```python
from build123d import *

# Parameters (mm, degrees)
ESQUISSE1_W                                    = 100
ESQUISSE1_H                                    = 100
ESQUISSE1_W_2                                  = 56.4
ESQUISSE1_H_2                                  = 56.4
BOSS_EXTRU_1_DEPTH                             = 10
CONG_1_R                                       = 3.2
BOSS_EXTRU_2_START                             = 10
ESQUISSE3_R                                    = 40
BOSS_EXTRU_2_DEPTH                             = 10
ESQUISSE4_OUTSIDE_W                            = 130.566
ESQUISSE4_OUTSIDE_H                            = 130.566
ESQUISSE4_OUTSIDE_R                            = 43
ENL_V_MAT_EXTRU_2_DEPTH                        = 0.5
ESQUISSE5_W                                    = 61.6
ESQUISSE5_H                                    = 61.6
ENL_V_MAT_EXTRU_3_DEPTH                        = 9
ESQUISSE6_W                                    = 61.6
ESQUISSE6_H                                    = 61.6
BOSS_EXTRU_3_DEPTH                             = 1
ESQUISSE12_W                                   = 100
ESQUISSE12_H                                   = 9.5
BOSS_EXTRU_5_DEPTH                             = 20
FRAISAGE_POUR_VIS_T_TE_FRAIS_E_M61_D           = 6.6
FRAISAGE_POUR_VIS_T_TE_FRAIS_E_M61_CSINK_D     = 12.6
FRAISAGE_POUR_VIS_T_TE_FRAIS_E_M61_CSINK_ANGLE = 90
ESQUISSE16_W                                   = 2
ESQUISSE16_H                                   = 10
ENL_V_MAT_EXTRU_4_DEPTH                        = 8
CONG_3_R                                       = 3.5
ESQUISSE17_W                                   = 10
ESQUISSE17_H                                   = 5
ENL_V_MAT_EXTRU_5_DEPTH                        = 89.317608663
CONG_4_R                                       = 3.5
CONG_5_R                                       = 3.3
CONG_6_R                                       = 4


with BuildPart() as part:
    # Esquisse1 → Boss.-Extru.1 (new body)
    with BuildSketch(Plane.XY):
        Rectangle(ESQUISSE1_W, ESQUISSE1_H)
        Rectangle(ESQUISSE1_W_2, ESQUISSE1_H_2, mode=Mode.SUBTRACT)
    extrude(amount=BOSS_EXTRU_1_DEPTH)

    # Congé1
    cong_1_edges = [part.edges().sort_by_distance(p)[0] for p in [
        (-28.2, 28.2, 5),
        (-28.2, -28.2, 5),
        (28.2, -28.2, 5),
        (28.2, 28.2, 5),
    ]]
    fillet(cong_1_edges, radius=CONG_1_R)

    # Esquisse3 → Boss.-Extru.2 (add)
    with BuildSketch(Plane.XY.offset(10).offset(BOSS_EXTRU_2_START)):
        Circle(ESQUISSE3_R)
        with BuildLine():
            Line((-28.2, 25), (-28.2, -25))
            ThreePointArc((-28.2, -25), (-27.2627417, -27.2627417), (-25, -28.2))
            Line((-25, -28.2), (25, -28.2))
            ThreePointArc((25, -28.2), (27.2627417, -27.2627417), (28.2, -25))
            Line((28.2, -25), (28.2, 25))
            ThreePointArc((28.2, 25), (27.2627417, 27.2627417), (25, 28.2))
            Line((25, 28.2), (-25, 28.2))
            ThreePointArc((-25, 28.2), (-27.2627417, 27.2627417), (-28.2, 25))
        make_face(mode=Mode.SUBTRACT)
    extrude(amount=-BOSS_EXTRU_2_DEPTH)

    # Esquisse4 outside → Enlèv. mat.-Extru.2 (cut)
    with BuildSketch(Plane.XY.offset(10)):
        Rectangle(ESQUISSE4_OUTSIDE_W, ESQUISSE4_OUTSIDE_H)
        Circle(ESQUISSE4_OUTSIDE_R, mode=Mode.SUBTRACT)
    extrude(amount=-ENL_V_MAT_EXTRU_2_DEPTH, mode=Mode.SUBTRACT)

    # Esquisse5 → Enlèv. mat.-Extru.3 (cut)
    with BuildSketch(Plane(origin=(0, 0, 0), x_dir=(-1, 0, 0), z_dir=(0, 0, -1))):
        Rectangle(ESQUISSE5_W, ESQUISSE5_H)
    extrude(amount=-ENL_V_MAT_EXTRU_3_DEPTH, mode=Mode.SUBTRACT)

    # Esquisse6 → Boss.-Extru.3 (add)
    with BuildSketch(Plane(origin=(0, 0, 9), x_dir=(-1, 0, 0), z_dir=(0, 0, -1))):
        Rectangle(ESQUISSE6_W, ESQUISSE6_H)
        with BuildLine():
            Line((28.2, -25), (28.2, 25))
            ThreePointArc((28.2, 25), (27.2627417, 27.2627417), (25, 28.2))
            Line((25, 28.2), (-25, 28.2))
            ThreePointArc((-25, 28.2), (-27.2627417, 27.2627417), (-28.2, 25))
            Line((-28.2, 25), (-28.2, -25))
            ThreePointArc((-28.2, -25), (-27.2627417, -27.2627417), (-25, -28.2))
            Line((-25, -28.2), (25, -28.2))
            ThreePointArc((25, -28.2), (27.2627417, -27.2627417), (28.2, -25))
        make_face(mode=Mode.SUBTRACT)
    extrude(amount=BOSS_EXTRU_3_DEPTH)

    # Esquisse12 → Boss.-Extru.5 (add)
    with BuildSketch(Plane.XZ.offset(50)):
        with Locations((0, 4.75)):
            Rectangle(ESQUISSE12_W, ESQUISSE12_H)
    extrude(amount=BOSS_EXTRU_5_DEPTH)

    # Fraisage pour vis à tête fraisée M61 (through all)
    with Locations(Plane(origin=(-40, -62, 9.5), x_dir=(1, 0, 0), z_dir=(0, 0, 1))):
        with Locations((0, 0), (20, 0), (40, 0), (60, 0), (80, 0), (0, 104), (80, 104)):
            CounterSinkHole(FRAISAGE_POUR_VIS_T_TE_FRAIS_E_M61_D / 2, FRAISAGE_POUR_VIS_T_TE_FRAIS_E_M61_CSINK_D / 2, counter_sink_angle=FRAISAGE_POUR_VIS_T_TE_FRAIS_E_M61_CSINK_ANGLE)

    # Esquisse16 → Enlèv. mat.-Extru.4 (cut)
    with BuildSketch(Plane(origin=(0, 0, 0), x_dir=(-1, 0, 0), z_dir=(0, 0, -1))):
        with Locations((31.8, 10.8)):
            Rectangle(ESQUISSE16_W, ESQUISSE16_H)
        with Locations((-31.8, -10.8)):
            Rectangle(ESQUISSE16_W, ESQUISSE16_H)
    extrude(amount=-ENL_V_MAT_EXTRU_4_DEPTH, mode=Mode.SUBTRACT)

    # Congé3
    # the kernel refuses this fillet: 3.5 mm, written as the material it adds along each edge
    with BuildSketch(Plane(origin=(32.8, -5.8, 0), x_dir=(-1, 0, 0), z_dir=(0, 0, 1)), Plane(origin=(-32.8, 5.8, 0), x_dir=(1, 0, 0), z_dir=(0, 0, 1))) as cong_3_piece_1:
        with BuildLine():
            CenterArc((3.5, 3.16227766), CONG_3_R, 180, 64.623066475)
            Line((0, 3.16227766), (-0.07, 3.16227766))
            Line((-0.07, 3.16227766), (-0.07, 0))
            Line((-0.07, 0), (0, -0.07))
            ThreePointArc((0, -0.07), (1, -0.07), (1.97, -0.063245553))
            Line((1.97, -0.063245553), (2, 0))
        make_face()
    extrude(amount=15.90569415)
    with BuildSketch(Plane(origin=(32.8, -15.8, 0), x_dir=(-1, 0, 0), z_dir=(0, 0, 1)), Plane(origin=(-32.8, 15.8, 0), x_dir=(1, 0, 0), z_dir=(0, 0, 1))) as cong_3_piece_2:
        with BuildLine():
            CenterArc((3.5, -3.16227766), CONG_3_R, 115.376933525, 64.623066475)
            Line((0, -3.16227766), (-0.07, -3.16227766))
            Line((-0.07, -3.16227766), (-0.07, 0))
            Line((-0.07, 0), (0, 0.07))
            ThreePointArc((0, 0.07), (1, 0.07), (1.97, 0.063245553))
            Line((1.97, 0.063245553), (2, 0))
        make_face()
    extrude(amount=15.90569415)

    # Esquisse17 → Enlèv. mat.-Extru.5 (cut, through all)
    with BuildSketch(Plane.XY.offset(20)):
        with Locations((0, -30.7)):
            Rectangle(ESQUISSE17_W, ESQUISSE17_H)
    extrude(amount=-ENL_V_MAT_EXTRU_5_DEPTH, mode=Mode.SUBTRACT)

    # Congé4
    cong_4_edges = [part.edges().sort_by_distance(p)[0] for p in [
        (5, -33.2, 10),
        (-5, -33.2, 10),
    ]]
    fillet(cong_4_edges, radius=CONG_4_R)

    # Congé5
    # the kernel refuses this fillet: 3.3 mm, written as the material it takes off along each edge
    with BuildSketch(Plane(origin=(-30.8, 5.8, -4.135900428), x_dir=(0, -1, 0), z_dir=(0, 0, 1))) as cong_5_piece_1:
        with BuildLine():
            CenterArc((1.654360171, -3.3), CONG_5_R, 90, 45.099127844)
            ThreePointArc((-0.683125835, -0.970588235), (-0.300120774, -0.514462201), (0, 0))
            Line((0, 0), (1.654360171, 0))
        make_face()
    extrude(amount=12.135900428, mode=Mode.SUBTRACT)
    with BuildSketch(Plane(origin=(-30.8, 15.8, -4.135900428), x_dir=(0, 1, 0), z_dir=(0, 0, 1)), Plane(origin=(30.8, -15.8, -4.135900428), x_dir=(0, -1, 0), z_dir=(0, 0, 1))) as cong_5_piece_2:
        with BuildLine():
            CenterArc((1.654360171, 3.3), CONG_5_R, 224.900872156, 45.099127844)
            ThreePointArc((-0.683125835, 0.970588235), (-0.300120774, 0.514462201), (0, 0))
            Line((0, 0), (1.654360171, 0))
        make_face()
    extrude(amount=12.135900428, mode=Mode.SUBTRACT)
    with BuildSketch(Plane(origin=(30.8, -5.8, -4.135900428), x_dir=(0.8177591102711759, -0.5755606289249594, 0), z_dir=(0, 0, 1))) as cong_5_piece_3:
        with BuildLine():
            CenterArc((1.746420483, 3.252218177), CONG_5_R, 215.138902841, 45.099127844)
            Line((-0.952184581, 1.352868102), (0, 0))
            ThreePointArc((0, 0), (0.593443854, 0.050677691), (1.186887707, 0))
        make_face()
    extrude(amount=12.135900428, mode=Mode.SUBTRACT)
    with BuildSketch(Plane(origin=(5, -28.2, 27.643596311), x_dir=(-0.0513844627897584, -0.9986789458999363, 0), z_dir=(0, 0, -1))) as cong_5_piece_4:
        with BuildLine():
            CenterArc((3.138535685, -3.22296821), CONG_5_R, 102.404067037, 74.650522983)
            Line((-0.157104836, -3.053399483), (-0.486668888, -3.03644261))
            Line((-0.486668888, -3.03644261), (-0.329564052, 0.016956873))
            Line((-0.329564052, 0.016956873), (0.016956873, 0.329564052))
            ThreePointArc((0.016956873, 0.329564052), (1.514975292, 0.252487358), (2.358794792, 0.322296821))
            Line((2.358794792, 0.322296821), (2.429680327, 0))
        make_face()
    extrude(amount=27.287192622, mode=Mode.SUBTRACT)
    with BuildSketch(Plane(origin=(-5, -28.2, 27.643596311), x_dir=(0.05138446278975914, -0.9986789458999363, 0), z_dir=(0, 0, -1))) as cong_5_piece_5:
        with BuildLine():
            CenterArc((3.138535685, 3.22296821), CONG_5_R, 182.94540998, 74.650522983)
            Line((-0.157104836, 3.053399483), (-0.486668888, 3.03644261))
            Line((-0.486668888, 3.03644261), (-0.329564052, -0.016956873))
            Line((-0.329564052, -0.016956873), (0.016956873, -0.329564052))
            ThreePointArc((0.016956873, -0.329564052), (1.514975292, -0.252487358), (2.358794792, -0.322296821))
            Line((2.358794792, -0.322296821), (2.429680327, 0))
        make_face()
    extrude(amount=27.287192622, mode=Mode.SUBTRACT)
    with BuildSketch(Plane(origin=(4.822649545, -30.8, 8), x_dir=(1, 0, 0), z_dir=(0, 0, -1))) as cong_5_piece_6:
        with BuildLine():
            CenterArc((1.861943014, 3.3), CONG_5_R, 220.32021507, 49.67978493)
            ThreePointArc((-0.654109258, 1.164705882), (-0.270973964, 0.613848345), (0, 0))
            Line((0, 0), (1.861943014, 0))
        make_face()
    extrude(amount=12.654857534, mode=Mode.SUBTRACT)
    with BuildSketch(Plane(origin=(-4.822649545, -30.8, -4.654857534), x_dir=(0.4896709556510413, -0.8719073088303573, 0), z_dir=(0, 0, 1))) as cong_5_piece_7:
        with BuildLine():
            CenterArc((1.965554704, -3.239355876), CONG_5_R, 101.001258329, 49.67978493)
            Line((-0.911739415, -1.623441722), (0, 0))
            ThreePointArc((0, 0), (0.667906938, -0.064319526), (1.335813877, 0))
        make_face()
    extrude(amount=12.654857534, mode=Mode.SUBTRACT)

    # Congé6
    cong_6_edges = [part.edges().sort_by_distance(p)[0] for p in [
        (-30.8, -30.8, 4),
        (30.8, -30.8, 4),
        (-30.8, 30.8, 4),
        (30.8, 30.8, 4),
    ]]
    fillet(cong_6_edges, radius=CONG_6_R)


solid = part.part
```
Work out the finished part from the listing and answer in its coordinate system (mm). A direction names the side the tool comes from. Give positions to 0.01 mm unless a question says otherwise; leave off trailing zeros. Write each loop counter-clockwise with the first axis right and the second up, starting at its lowest first coordinate (ties: lowest second). Pieces come first, ordered by that corner, then holes.
(1) The part is cut by section A-A on y = -62. Count the separate pieces of the cut face and the enclosed holes in it, plus the area to 4 significant figures.
Final values:
separate pieces: 6
enclosed holes: 0
area: 591.5 mm2
(2) The part is cut by section D-D on x = -10. Write down the section's boundary in (y, z), plus the area to 3 significant figures.
Final values:
outline: (-70, 0) - (-30.8, 0) - (-30.8, 8) - (-28.2, 8) - (-28.2, 20) - (-38.73, 20) - (-38.73, 10) - (-41.82, 10) - (-41.82, 9.5) - (-70, 9.5) - close; (28.2, 8) - (30.8, 8) - (30.8, 0) - (50, 0) - (50, 9.5) - (41.82, 9.5) - (41.82, 10) - (38.73, 10) - (38.73, 20) - (28.2, 20) - close
area: 787 mm2
(3) Flat-ended cylindrical pins translate along their axes: pin 1 Ø3 at (x, z) = (15.5, 13) entering from -Y; pin 2 Ø8.5 at (x, y) = (-40, -62) entering from +Z; pin 3 Ø5.5 at (x, y) = (20, -62) entering from +Z; pin 4 Ø3 at (x, y) = (-21, -54.5) entering from +Z. Find the tip coordinate at first contact, or state that the pin passes through.
Final values:
pin 1: stops at y = -37.47
pin 2: stops at z = 7.45
pin 3: passes through
pin 4: stops at z = 9.5
(4) The part is cut by section B-B on x = 0. Write down the section's boundary in (y, z), plus the area to 4 significant figures.
Final values:
outline: (-70, 0) - (-65.3, 0) - (-65.3, 6.5) - (-68.3, 9.5) - (-70, 9.5) - close; (-58.7, 0) - (-33.2, 0) - (-33.2, 20) - (-40, 20) - (-40, 10) - (-43, 10) - (-43, 9.5) - (-55.7, 9.5) - (-58.7, 6.5) - close; (28.2, 8) - (30.8, 8) - (30.8, 0) - (50, 0) - (50, 9.5) - (43, 9.5) - (43, 10) - (40, 10) - (40, 20) - (28.2, 20) - close
area: 662.5 mm2
(5) The part is cut by section C-C on z = 17.5. Write down the section's boundary in (x, y), plus the area to 3 significant figures.
Final values:
outline: circle Ø80 at (0, 0); hole (-28.2, -25) arc R3.2 ccw to (-25, -28.2) - (-8.06, -28.2) arc R3.3 cw to (-4.88, -30.63) arc R3.5 ccw to (-1.5, -33.2) - (1.5, -33.2) arc R3.5 ccw to (4.88, -30.63) arc R3.3 cw to (8.06, -28.2) - (25, -28.2) arc R3.2 ccw to (28.2, -25) - (28.2, 25) arc R3.2 ccw to (25, 28.2) - (-25, 28.2) arc R3.2 ccw to (-28.2, 25) - close
area: 1,810 mm2
(6) Straight lines are drawn through the part: line 1 (Y direction, x = -20, z = 2.5); line 2 (Y direction, x = 0, z = 3.5); line 3 (X direction, y = -62, z = 4.75). For each, find the intervals that lie inside material, in ascending order.
Final values:
line 1: y = -70 to -65.3, -58.7 to -30.8, 30.8 to 50
line 2: y = -70 to -65.3, -58.7 to -33.2, 30.8 to 50
line 3: x = -50 to -43.3, -36.7 to -23.3, -16.7 to -3.3, 3.3 to 16.7, 23.3 to 36.7, 43.3 to 50
(7) Which of the six approach directions +Z, -Z, +X, -X, +Y, -Y give full straight-line access (tool end or side, diameter ignored) to faces 1 (the flat face through (17, -28.2, 14)), 2 (the cylindrical face through (29.659, -29.597, 4.056)), 3 (the flat face through (-1, -38, 0))?
Final values:
face 1: +Z, -Z
face 2: -Z
face 3: -Z, +X, -X, +Y, -Y
(8) The mould has two halves that part along X. Classify faces 4 (the flat face through (-1, 50, 5)), 5 (the flat face through (0, -33.2, 10)): pulls with the +X half, pulls with the -X half, needs draft (parallel to the pull), parting line crosses it, or undercut.
Final values:
face 4: needs draft
face 5: undercut
